```python
from build123d import *
from OCP.BRepFilletAPI import BRepFilletAPI_MakeFillet

# Parameters (mm, degrees)
SCHIZZO1_R                     = 37.5
FISSAGGIOMANDRINO_DEPTH        = 25
SCHIZZO2_W                     = 120
SCHIZZO2_H                     = 100
PIASTRA_DEPTH                  = 20
SCHIZZO3_R                     = 3.125
ACCOPPIAMENTOMANDRINI_DEPTH    = 7
SCHIZZO4_W                     = 20
SCHIZZO4_H                     = 100
BASEADATTATORE_DEPTH           = 150
RACCORDO1_R                    = 20
SCHIZZO5_W                     = 70
SCHIZZO5_H                     = 75
BASETORCIA_DEPTH               = 37.5
SCHIZZO6_R                     = 25
FOROTORICA_DEPTH               = 183.002747232
SCHIZZO7_R                     = 25
SCHIZZO7_R_2                   = 22.5
CONTATTOPOSTERIORETORCIA_DEPTH = 5
SCHIZZO8_R                     = 25
SCHIZZO8_R_2                   = 23
PRIMOCONTATTOANTERIORE_DEPTH   = 2
SCHIZZO9_R                     = 25
SCHIZZO9_R_2                   = 20
SECONDOCONTATTOANTERIORE_DEPTH = 4
RACCORDO2_R1                   = 20
RACCORDO2_R2                   = 6


with BuildPart() as part:
    # Schizzo1 → FissaggioMandrino (new body)
    with BuildSketch(Plane.XY):
        Circle(SCHIZZO1_R)
    extrude(amount=-FISSAGGIOMANDRINO_DEPTH)

    # Schizzo2 → Piastra (add)
    with BuildSketch(Plane.XY):
        with Locations((-10, 0)):
            Rectangle(SCHIZZO2_W, SCHIZZO2_H)
    extrude(amount=PIASTRA_DEPTH)

    # Schizzo3 → AccoppiamentoMandrini (cut)
    with BuildSketch(Plane(origin=(0, 0, -25), x_dir=(-1, 0, 0), z_dir=(0, 0, -1))):
        with Locations((29.375, 0)):
            Circle(SCHIZZO3_R)
        with Locations((27.138961268, -11.241325826)):
            Circle(SCHIZZO3_R)
        with Locations((20.771261697, -20.771261697)):
            Circle(SCHIZZO3_R)
        with Locations((11.241325826, -27.138961268)):
            Circle(SCHIZZO3_R)
        with Locations((0, -29.375)):
            Circle(SCHIZZO3_R)
        with Locations((-11.241325826, -27.138961268)):
            Circle(SCHIZZO3_R)
        with Locations((-20.771261697, -20.771261697)):
            Circle(SCHIZZO3_R)
        with Locations((-27.138961268, -11.241325826)):
            Circle(SCHIZZO3_R)
        with Locations((-29.375, 0)):
            Circle(SCHIZZO3_R)
        with Locations((-27.138961268, 11.241325826)):
            Circle(SCHIZZO3_R)
        with Locations((-20.771261697, 20.771261697)):
            Circle(SCHIZZO3_R)
        with Locations((-11.241325826, 27.138961268)):
            Circle(SCHIZZO3_R)
        with Locations((0, 29.375)):
            Circle(SCHIZZO3_R)
        with Locations((11.241325826, 27.138961268)):
            Circle(SCHIZZO3_R)
        with Locations((20.771261697, 20.771261697)):
            Circle(SCHIZZO3_R)
        with Locations((27.138961268, 11.241325826)):
            Circle(SCHIZZO3_R)
    extrude(amount=-ACCOPPIAMENTOMANDRINI_DEPTH, mode=Mode.SUBTRACT)

    # Schizzo4 → BaseAdattatore (add)
    with BuildSketch(Plane.XY.offset(20)):
        with Locations((-60, 0)):
            Rectangle(SCHIZZO4_W, SCHIZZO4_H)
    extrude(amount=BASEADATTATORE_DEPTH)

    # Raccordo1
    raccordo1_edges = [part.edges().sort_by_distance(p)[0] for p in [
        (-70, 0, 0),
        (50, -50, 10),
        (50, 50, 10),
        (-50, 0, 20),
        (-60, -50, 170),
        (-60, 50, 170),
    ]]
    fillet(raccordo1_edges, radius=RACCORDO1_R)

    # Schizzo5 → BaseTorcia (add, symmetric)
    with BuildSketch(Plane(origin=(0, 0, 0), x_dir=(1, 0, 0), z_dir=(0, 1, 0))):
        with Locations((-105, -117.5)):
            Rectangle(SCHIZZO5_W, SCHIZZO5_H)
    extrude(amount=BASETORCIA_DEPTH, both=True)

    # Schizzo6 → ForoTorica (cut, through all)
    with BuildSketch(Plane(origin=(0, 0, 80), x_dir=(-1, 0, 0), z_dir=(0, 0, -1))):
        with Locations((105, 0)):
            Circle(SCHIZZO6_R)
    extrude(amount=-FOROTORICA_DEPTH, mode=Mode.SUBTRACT)

    # Schizzo7 → ContattoPosterioreTorcia (add)
    with BuildSketch(Plane(origin=(0, 0, 80), x_dir=(-1, 0, 0), z_dir=(0, 0, -1))):
        with Locations((105, 0)):
            Circle(SCHIZZO7_R)
        with Locations((105, 0)):
            Circle(SCHIZZO7_R_2, mode=Mode.SUBTRACT)
    extrude(amount=-CONTATTOPOSTERIORETORCIA_DEPTH)

    # Schizzo8 → PrimoContattoAnteriore (add)
    with BuildSketch(Plane.XY.offset(149)):
        with Locations(Location((-105, 0, 0), (0, 0, 180))):
            Circle(SCHIZZO8_R)
        with Locations((-105, 0)):
            Circle(SCHIZZO8_R_2, mode=Mode.SUBTRACT)
    extrude(amount=PRIMOCONTATTOANTERIORE_DEPTH)

    # Schizzo9 → SecondocontattoAnteriore (add)
    with BuildSketch(Plane.XY.offset(151)):
        with Locations(Location((-105, 0, 0), (0, 0, 180))):
            Circle(SCHIZZO9_R)
        with Locations(Location((-105, 0, 0), (0, 0, 180))):
            Circle(SCHIZZO9_R_2, mode=Mode.SUBTRACT)
    extrude(amount=SECONDOCONTATTOANTERIORE_DEPTH)

    # Raccordo2: one fillet with a radius per group of edges: ONE call of the kernel's fillet builder (fillet() takes one radius for all edges)
    raccordo2_edges_1 = [part.edges().sort_by_distance(p)[0] for p in [
        (-140, -37.5, 117.5),
        (-140, 37.5, 117.5),
    ]]
    raccordo2_edges_2 = [part.edges().sort_by_distance(p)[0] for p in [
        (-70, 37.5, 117.5),
        (-70, -37.5, 117.5),
        (-70, 0, 80),
        (-70, 0, 155),
    ]]
    raccordo2 = BRepFilletAPI_MakeFillet(part.part.solid().wrapped)
    for e in raccordo2_edges_1:
        raccordo2.Add(RACCORDO2_R1, e.wrapped)
    for e in raccordo2_edges_2:
        raccordo2.Add(RACCORDO2_R2, e.wrapped)
    add(Compound.cast(raccordo2.Shape()), mode=Mode.REPLACE)


solid = part.part
```
Build history of the part. All positions in model axes, mm. A direction names the side the tool comes from. Coordinates: 2 decimals unless noted, no trailing zeros. Write each loop counter-clockwise with the first axis right and the second up, starting at its lowest first coordinate (ties: lowest second). Pieces come first, ordered by that corner, then holes.
1. Band-saw the part on B-B, the plane x = -105. Give the cut face in (y, z), and give its area (3 significant figures).
Answer block:
outline: (-37.5, 80) - (-22.5, 80) - (-22.5, 85) - (-25, 85) - (-25, 149) - (-23, 149) - (-23, 151) - (-20, 151) - (-20, 155) - (-37.5, 155) - close; (20, 151) - (23, 151) - (23, 149) - (25, 149) - (25, 85) - (22.5, 85) - (22.5, 80) - (37.5, 80) - (37.5, 155) - (20, 155) - close
area: 1,950 mm2
2. 3-axis set-ups, long thin cutter, end or side, ignore diameter. For faces 1 (the flat face through (50, 0, 10)), 2 (the cylindrical face through (-32.356, 0.939, -21.549)), 3 (the flat face through (-98, 37.5, 117)): which of +Z, -Z, +X, -X, +Y, -Y reach the whole face in a straight line?
Answer block:
face 1: +Z, -Z, +X, +Y, -Y
face 2: -Z
face 3: +Z, -Z, -X, +Y
3. Drill centre lines: probe 1 along X at (y, z) = (-1, 106.5); probe 2 along X at (y, z) = (-22, 110.5); probe 3 along Z at (x, y) = (-80, -30). Where is each one in solid material? Low to high.
Answer block:
probe 1: x = -140 to -129.98, -80.02 to -50
probe 2: x = -139.49 to -116.87, -93.13 to -50
probe 3: z = 80 to 155
4. Band-saw the part on D-D, the plane z = -12.5. Give the cut face in (x, y), and give its area (3 significant figures).
Answer block:
outline: circle Ø75 at (0, 0)
area: 4,420 mm2
5. Pull direction Y, two halves, no side cores. Call faces 4 (the cylindrical face through (-22.451, -18.136, -21.549)), 5 (the cylindrical face through (44.297, 43.986, 10.14)), 6 (the flat face through (-98, -37.5, 117)): released by +Y, released by -Y, zero draft, split by the parting line, or undercut.
Answer block:
face 4: undercut
face 5: released by +Y
face 6: released by -Y
6. Band-saw the part on A-A, the plane z = 131.5. Give the cut face in (x, y), and give its area (3 significant figures).
Answer block:
outline: (-140, -17.5) arc R20 ccw to (-120, -37.5) - (-76, -37.5) arc R6 cw to (-70, -43.5) - (-70, -50) - (-50, -50) - (-50, 50) - (-70, 50) - (-70, 43.5) arc R6 cw to (-76, 37.5) - (-120, 37.5) arc R20 ccw to (-140, 17.5) - close; hole circle Ø50 at (-105, 0)
area: 5,130 mm2
7. Band-saw the part on C-C, the plane x = 0. Give the cut face in (y, z).
Answer block:
outline: (-50, 0) - (-37.5, 0) - (-37.5, -25) - (-32.5, -25) - (-32.5, -18) - (-26.25, -18) - (-26.25, -25) - (26.25, -25) - (26.25, -18) - (32.5, -18) - (32.5, -25) - (37.5, -25) - (37.5, 0) - (50, 0) - (50, 20) - (-50, 20) - close
8. Drop flat-ended pins along their axis: pin 1 (1.9 mm diameter, centred on x = -27.5, y = -11.5, fed in from -Z); pin 2 (6 mm diameter, centred on x = -30, y = 20.5, fed in from +Z); pin 3 (3 mm diameter, centred on x = 20.5, y = -22.5, fed in from -Z); pin 4 (1 mm diameter, centred on y = -4, z = 31.5, fed in from +X). Give the stop position or say it passes through.
Answer block:
pin 1: stops at z = -18
pin 2: stops at z = 20.23
pin 3: stops at z = -25
pin 4: stops at x = -47.86
